Read the model definition and answer for the solid it produces. Units are mm, in the model's axes. Face numbers are marked on the shaded views. A direction names the side the tool comes from. Give positions to 0.01 mm unless a question says otherwise; leave off trailing zeros. Write each loop counter-clockwise with the first axis right and the second up, starting at its lowest first coordinate (ties: lowest second). Pieces come first, ordered by that corner, then holes. Notation, with made-up numbers: (17.5, 5) - (72.5, 5) arc R16 ccw to (72.5, 14) - close; hole circle Ø4 at (29.25, 71). An arc over 180 degrees is marked (long way). Answer as CSV lines item,"result".
```python
from build123d import *

# Parameters (mm, degrees)
SKETCH022_W            = 190
SKETCH022_H            = 95
PAD014_DEPTH           = 5
SKETCH023_W            = 3
SKETCH023_H            = 20
PAD015_DEPTH           = 60
LINEARPATTERN009_COUNT = 8
LINEARPATTERN009_PITCH = 22.142857


with BuildPart() as part:
    # Sketch022 → Pad014 (new body)
    with BuildSketch(Plane.XY):
        Rectangle(SKETCH022_W, SKETCH022_H)
    extrude(amount=PAD014_DEPTH)

    # Sketch023 (on DatumPlane) → Pad015 (join)
    with BuildSketch(Plane(origin=(62, 0, 4), x_dir=(0.866025, 0, -0.5), z_dir=(0.5, 0, 0.866025))):
        with Locations((0, 30)):
            Rectangle(SKETCH023_W, SKETCH023_H)
        with Locations((0, -30)):
            Rectangle(SKETCH023_W, SKETCH023_H)
    pad015 = extrude(amount=PAD015_DEPTH)

    # LinearPattern009: Pad015 ×8
    with Locations(*[(-i * LINEARPATTERN009_PITCH, 0, 0) for i in range(1, LINEARPATTERN009_COUNT)]):
        add(pad015)


with BuildPart() as part_1:
    # Body007 placement: moved
    add(part.part.moved(Location((0, 132, 0))))


solid = part_1.part
```
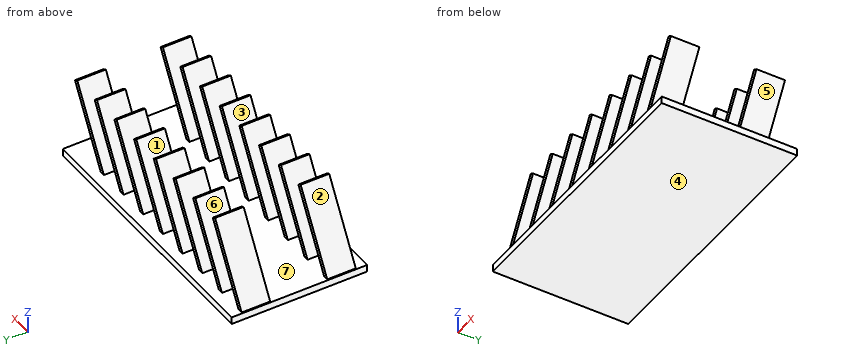
(1) The mould has two halves that part along Z. Classify the marked faces 1, 2, 3 and 4: +Z half, -Z half, draft (parallel to the pull), parting line (faces both ways), or undercut.
Worked out:
face 1,"undercut"
face 2,"+Z half"
face 3,"undercut"
face 4,"-Z half"
(2) A cutting plane is placed at A-A (x = 29.5). Write down the section's boundary in (y, z).
Worked out:
outline,"(84.5, 0) - (179.5, 0) - (179.5, 5) - (84.5, 5) - close; (92, 21.41) - (112, 21.41) - (112, 27.41) - (92, 27.41) - close; (152, 21.41) - (172, 21.41) - (172, 27.41) - (152, 27.41) - close"
(3) A cutting plane is placed at C-C (z = 35.5). Count the separate pieces of the cut face and the enclosed holes in it, and give its area (3 significant figures).
Worked out:
separate pieces,"16"
enclosed holes,"0"
area,"1,110 mm^2"
(4) A cutting plane is placed at B-B (y = 125.5). Write down the section's boundary in (x, z), and give its area (3 significant figures).
Worked out:
outline,"(-95, 0) - (95, 0) - (95, 5) - (-95, 5) - close"
area,"950 mm^2"
(5) For the marked faces 5, 6 and 7, determine the directions among +Z, -Z, +X, -X, +Y, -Y from which every point of the face is accessible in a straight line to the end or side of a thin tool.
Worked out:
face 5,"+X, +Y, -Y"
face 6,"+Y, -Y"
face 7,"none"
(6) Find the intervals of material crossed by L1, parallel to Y at x = 63.5, z = 9; L2, parallel to Z at x = -23, y = 168; L3, parallel to Z at x = 8, y = 115, in increasing order.
Worked out:
L1,"y = 92 to 112, 152 to 172"
L2,"z = 0 to 5, 7.19 to 13.19, 45.54 to 51.54"
L3,"z = 0 to 5"
(7) Each of these flat-tipped pins is pushed along its axis until it touches: P1, Ø3, axis at y = 103, z = 35, coming from the +X side; P2, Ø12, axis at y = 159.5, z = 40, coming from the -X side; P3, Ø16, axis at x = -85, z = 41.5, coming from the +Y side; P4, Ø10, axis at x = -18, y = 105, coming from the +Z side. Where does it stop, or does it pass through?
Worked out:
P1,"stops at x = 82.5"
P2,"stops at x = -77.41"
P3,"passes through"
P4,"stops at z = 56.71"
